Autodesk Inventor part; units mm, degrees
ref_plane "YZ Plane" through (0, 0, 0) normal (1, 0, 0) x (0, 1, 0)
ref_plane "XZ Plane" through (0, 0, 0) normal (0, 1, 0) x (-1, 0, 0)
ref_plane "XY Plane" through (0, 0, 0) normal (0, 0, 1) x (1, 0, 0)
sketch "Szkic1" plane through (0, 0, 0) normal (0, 1, 0) x (-1, 0, 0)
  circle A0 centre (0, 0) radius 15
  arc A1 (3.6, 1.575) -> (3.6, -1.575) centre (1.5, 0) ccw
  line L0 (3.6, -1.575) -> (3.6, 1.575)
  dimension "d0" = 30
  dimension "d1" = 5.25
  dimension "d2" = 3.6
extrude "Wyciągnięcie proste1" add sketch "Szkic1" along normal blind 20
sketch "Szkic2" plane through (0, 20, 0) normal (0, 1, 0) x (1, 0, 0)
  circle A0 centre (0, 0) radius 15
  circle A1 centre (0, 0) radius 12.5
extrude "Wyciągnięcie proste2" add sketch "Szkic2" against normal blind 2 contours A0 | A1
sketch "Szkic3" plane through (0, 20, 0) normal (0, 1, 0) x (1, 0, 0)
  circle A0 centre (0, 0) radius 15
  circle A1 centre (0, 0) radius 12.5
  dimension "d7" = 25
extrude "Wyciągnięcie proste3" cut sketch "Szkic3" against normal blind 15
sketch "Szkic4" plane through (0, 20, 0) normal (0, 1, 0) x (1, 0, 0)
  circle A0 centre (0, 0) radius 10
  circle A1 centre (0, 0) radius 12.5
  dimension "d10" = 20
extrude "Wyciągnięcie proste4" cut sketch "Szkic4" against normal blind 6
sketch "Szkic5" plane through (0, 18, 0) normal (0, -1, 0) x (1, 0, 0)
  point P0 (0, 0)
sketch "Szkic6" plane through (0, 0, 0) normal (0, -1, 0) x (1, 0, 0)
  circle A0 centre (0, 0) radius 15
  line L0 (-3.6, 1.575) -> (-3.6, -1.575)
  line L1 (-3.6, 1.575) -> (-3.6, -1.575)
  arc A1 (-3.6, -1.575) -> (-3.6, 1.575) centre (-1.5, 0) ccw
extrude "Wyciągnięcie proste5" add sketch "Szkic6" along normal blind 2
properties part number "_Drukowanie 3D"
The listing builds one solid part. Answer for the finished solid, in the listing's coordinates (mm). A direction names the side the tool comes from. Round coordinates to 2 decimals unless told otherwise and drop trailing zeros. Loops run counter-clockwise (first coordinate to the right, second up) from the corner with the lowest first, then second, coordinate; pieces in that order, holes last. Notation, with made-up numbers: (62, 61) -> (112, 61) arc R26 cw to (112, 93) -> close; hole circle Ø1 at (50, 69.25). An arc over 180 degrees is marked (long way). Use one line per item in the form item = value.
1. Flat-ended cylindrical pins translate along their axes: pin 1 Ø12 at (x, y) = (2.5, 16.5) entering from +Z; pin 2 Ø4 at (x, y) = (8, 5) entering from +Z; pin 3 Ø2 at (x, y) = (-7, 12) entering from -Z. Find the tip coordinate at first contact, or state that the pin passes through.
Answer key:
pin_1 = 12.5
pin_2 = 13.75
pin_3 = -10.97
2. The part is cut by section D-D on y = 18.75. Determine the outline of the cut face in (x, z), and give its area (3 significant figures).
Answer key:
outline = circle Ø20 at (0, 0)
area = 314 mm²
3. The part is cut by section B-B on y = 9. Determine the outline of the cut face in (x, z) (3 decimals).
Answer key:
outline = circle Ø25 at (0, 0); hole (-3.6, -1.575) arc R2.625 ccw (long way) to (-3.6, 1.575) -> close
4. The part is cut by section A-A on z = 0. Determine the outline of the cut face in (x, y) (3 decimals), and give its area (4 significant figures).
Answer key:
outline = (-15, -2) -> (-3.6, -2) -> (-3.6, 18) -> (1.125, 18) -> (1.125, -2) -> (15, -2) -> (15, 5) -> (12.5, 5) -> (12.5, 14) -> (10, 14) -> (10, 20) -> (-10, 20) -> (-10, 14) -> (-12.5, 14) -> (-12.5, 5) -> (-15, 5) -> close
area = 460.5 mm²
5. For a pull along X with two mould halves and no side action, classify faces 4 (the cylindrical face through (-2.17, 17.04, 9.76)), 5 (the flat face through (-1, 18, 0)), 6 (the flat face through (0, 20, 0)) as released by +X, released by -X, zero draft, split by the parting line, or undercut.
Answer key:
face_4 = split by the parting line
face_5 = undercut
face_6 = zero draft
6. A tool of negligible diameter and unlimited length cuts with its end or side. For faces 1 (the cylindrical face through (1.123, 8.14, 0.092)), 2 (the flat face through (-0.1, 14, -10.2)), 3 (the flat face through (3, -2, 0)), from which of +Z, -Z, +X, -X, +Y, -Y can it reach the whole face along a straight path? Write none if from no direction.
Answer key:
face_1 = -Y
face_2 = +Y
face_3 = +Z, -Z, +X, -X, -Y
7. Find the intervals of material crossed by probe 1 along X at (y, z) = (6.5, 0) (3 decimals); probe 2 along X at (y, z) = (3.75, 0) (3 decimals); probe 3 along Y at (x, z) = (6.75, 8.5), in increasing order. Write a range as [from, to].
Answer key:
probe_1 = [-12.5, -3.6], [1.125, 12.5]
probe_2 = [-15, -3.6], [1.125, 15]
probe_3 = [-2, 14]
8. The part is cut by section C-C on x = -1.5. Determine the outline of the cut face in (y, z) (3 decimals).
Answer key:
outline = (-2, -14.925) -> (5, -14.925) -> (5, -12.41) -> (14, -12.41) -> (14, -9.887) -> (20, -9.887) -> (20, 9.887) -> (14, 9.887) -> (14, 12.41) -> (5, 12.41) -> (5, 14.925) -> (-2, 14.925) -> (-2, 2.625) -> (18, 2.625) -> (18, -2.625) -> (-2, -2.625) -> close
